Read the model definition and answer for the solid it produces. Units are mm, in the model's axes. Face numbers are marked on the shaded views. A direction names the side the tool comes from. Coordinates: 2 decimals unless noted, no trailing zeros. Loops run counter-clockwise (first coordinate to the right, second up) from the corner with the lowest first, then second, coordinate; pieces in that order, holes last.
Autodesk Inventor part; units mm, degrees
ref_plane "YZ Plane" through (0, 0, 0) normal (1, 0, 0) x (0, 1, 0)
ref_plane "XZ Plane" through (0, 0, 0) normal (0, 1, 0) x (-1, 0, 0)
ref_plane "XY Plane" through (0, 0, 0) normal (0, 0, 1) x (1, 0, 0)
sketch "Skizze1" plane through (0, 0, 0) normal (0, 0, 1) x (1, 0, 0)
  line L0 (-9.5, 13) -> (9.5, 13)
  line L1 (9.5, 13) -> (9.5, -13)
  line L2 (9.5, -13) -> (-9.5, -13)
  line L3 (-9.5, -13) -> (-9.5, 13)
  line L4 (-9.5, 13) -> (9.5, -13) construction
  line L5 (9.5, 13) -> (-9.5, -13) construction
  point P0 (0, 0)
  dimension "d0" = 19
  dimension "d1" = 26
extrude "Extrusion1" add sketch "Skizze1" along normal blind 8
sketch "Skizze2" plane through (0, 0, 8) normal (0, 0, 1) x (1, 0, 0)
  circle A0 centre (-1.1, -2.6) radius 3.5
  line L0 (-9.5, -13) -> (9.5, -13)
  line L1 (-9.5, 13) -> (-9.5, -13)
  point P0 (0, 0)
  dimension "d4" = 7
  dimension "d5" = 10.4
  dimension "d6" = 8.4
extrude "Extrusion2" add sketch "Skizze2" along normal blind 8
properties part number "encoder"
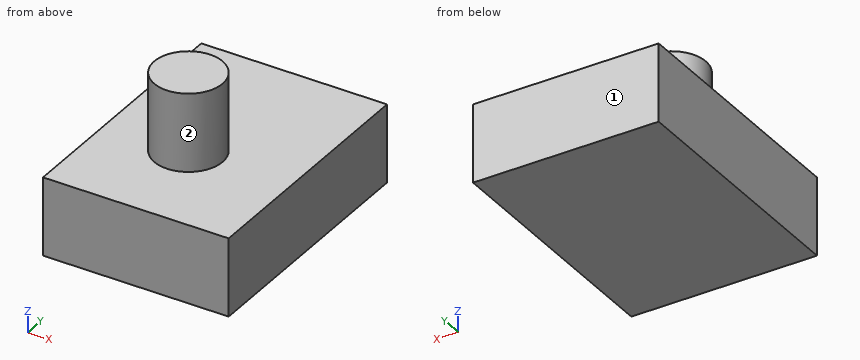
Q1. A flat-ended cylindrical pin translates along its axis: pin 1 Ø1.5 at (x, y) = (-4, -10) entering from +Z. Find the tip coordinate at first contact, or state that the pin passes through.
Findings below:
pin 1: stops at z = 8
Q2. A cutting plane is placed at D-D (y = -7.5). Give the vertices of the cut face in (x, z).
Findings below:
outline: (-9.5, 0) - (9.5, 0) - (9.5, 8) - (-9.5, 8) - close
Q3. A cutting plane is placed at A-A (y = -2.6). Give the vertices of the cut face in (x, z), then the cut area to 3 significant figures.
Findings below:
outline: (-9.5, 0) - (9.5, 0) - (9.5, 8) - (2.4, 8) - (2.4, 16) - (-4.6, 16) - (-4.6, 8) - (-9.5, 8) - close
area: 208 mm2
Q4. Straight lines are drawn through the part: probe 1 along Z at (x, y) = (-2.75, 7.5); probe 2 along Y at (x, z) = (-2.75, 15.25); probe 3 along Y at (x, z) = (-0.25, 15.25). For each, find the intervals that lie inside material, in ascending order.
Findings below:
probe 1: z = 0 to 8
probe 2: y = -5.69 to 0.49
probe 3: y = -6 to 0.8
Q5. Which of the six approach directions +Z, -Z, +X, -X, +Y, -Y give full straight-line access (tool end or side, diameter ignored) to the marked faces 1 and 2?
Findings below:
face 1: +Z, -Z, +X, -X, +Y
face 2: +Z
Q6. A cutting plane is placed at B-B (x = -1.1). Give the vertices of the cut face in (y, z), then the cut area to 3 significant figures.
Findings below:
outline: (-13, 0) - (13, 0) - (13, 8) - (0.9, 8) - (0.9, 16) - (-6.1, 16) - (-6.1, 8) - (-13, 8) - close
area: 264 mm2
Q7. A cutting plane is placed at C-C (z = 14.75). Give the vertices of the cut face in (x, y), then the cut area to 3 significant figures.
Findings below:
outline: circle Ø7 at (-1.1, -2.6)
area: 38.5 mm2
